from build123d import *

# Parameters (mm, degrees)
SKETCH_1_W             = 250
SKETCH_1_H             = 750
EXTRUDE_1_DEPTH        = 16
CUT_EXTRUDE_2_DEPTH    = 20
SKETCH_5_R             = 6.5
CUT_EXTRUDE_3_DEPTH    = 791.731307082
PATTERN_LINEAR_1_COUNT = 5
PATTERN_LINEAR_1_PITCH = 50
SKETCH_6_R             = 28
CUT_EXTRUDE_4_DEPTH    = 791.731307082
FILLET_1_R             = 60
SKETCH_7_W             = 250
SKETCH_7_H             = 40
CUT_EXTRUDE_5_DEPTH    = 66


with BuildPart() as part:
    # 草图1 → 凸台-拉伸1 (new body)
    with BuildSketch(Plane(origin=(0, 0, 0), x_dir=(0, 0, -1), z_dir=(1, 0, 0))):
        with Locations((125, 375)):
            Rectangle(SKETCH_1_W, SKETCH_1_H)
    extrude(amount=EXTRUDE_1_DEPTH)

    # 草图3 → 切除-拉伸2 (cut)
    with BuildSketch(Plane.ZY):
        Polygon((-130, 0), (0, 250), (0, 0), align=None)
    extrude(amount=-CUT_EXTRUDE_2_DEPTH, mode=Mode.SUBTRACT)

    # 草图5 → 切除-拉伸3 (cut, through all)
    with BuildSketch(Plane.ZY):
        with Locations((-225, 665)):
            Circle(SKETCH_5_R)
        with Locations((-225, 505)):
            Circle(SKETCH_5_R)
        with Locations((-225, 485)):
            Circle(SKETCH_5_R)
    cut_extrude_3 = extrude(amount=-CUT_EXTRUDE_3_DEPTH, mode=Mode.SUBTRACT)

    # 阵列(线性)1: 切除-拉伸3 ×5
    with Locations(*[(0, 0, i * PATTERN_LINEAR_1_PITCH) for i in range(1, PATTERN_LINEAR_1_COUNT)]):
        add(cut_extrude_3, mode=Mode.SUBTRACT)

    # 草图6 → 切除-拉伸4 (cut, through all)
    with BuildSketch(Plane.ZY):
        with Locations((-140, 105)):
            Circle(SKETCH_6_R)
    extrude(amount=-CUT_EXTRUDE_4_DEPTH, mode=Mode.SUBTRACT)

    # 圆角1
    fillet_1_edges = [part.edges().sort_by_distance(p)[0] for p in [
        (8, 0, -130),
        (8, 250, 0),
    ]]
    fillet(fillet_1_edges, radius=FILLET_1_R)

    # 草图7 → 切除-拉伸5 (cut)
    with BuildSketch(Plane(origin=(16, 0, 0), x_dir=(0, 0, -1), z_dir=(1, 0, 0))):
        with Locations((125, 730)):
            Rectangle(SKETCH_7_W, SKETCH_7_H)
    extrude(amount=-CUT_EXTRUDE_5_DEPTH, mode=Mode.SUBTRACT)


solid = part.part
Check sheet for the modelled part. Datum: model origin and axes. Units: mm. Coordinates: 2 decimals unless noted, no trailing zeros. Loops run counter-clockwise (first coordinate to the right, second up) from the corner with the lowest first, then second, coordinate; pieces in that order, holes last. Notation, with made-up numbers: (59, 87) -> (101, 87) arc R28 ccw to (101, 123) -> close; hole circle Ø3 at (57.25, 18). An arc over 180 degrees is marked (long way). Answer in a Markdown table with one row per item.
1. Sectioned sample at D-D, the plane z = -25. Record the boundary of the cut face in (x, y).
Check values:
| item | result |
|---|---|
| outline | (0, 201.92) -> (16, 201.92) -> (16, 478.5) -> (0, 478.5) -> close; (0, 491.5) -> (16, 491.5) -> (16, 498.5) -> (0, 498.5) -> close; (0, 511.5) -> (16, 511.5) -> (16, 658.5) -> (0, 658.5) -> close; (0, 671.5) -> (16, 671.5) -> (16, 710) -> (0, 710) -> close |
2. Release check for a two-part mould opening along Z. For faces 1 (the face through (8.112, 250.615, -1.669)), 2 (the face through (0, 360, -123)), 3 (the face through (7.888, 659.233, -72.001)) record: released by +Z, released by -Z, zero draft, split by the parting line, or undercut.
Check values:
| item | result |
|---|---|
| face 1 | released by +Z |
| face 2 | zero draft |
| face 3 | undercut |
3. Sectioned sample at B-B, the plane x = 3.75. Give the number of separate pieces and of enclosed holes in the cut face, then the cut area to 3 significant figures.
Check values:
| item | result |
|---|---|
| separate pieces | 1 |
| enclosed holes | 16 |
| area | 157,000 mm2 |
4. Sectioned sample at C-C, the plane y = 665. Record the boundary of the cut face in (x, z), then the cut area to 3 significant figures.
Check values:
| item | result |
|---|---|
| outline | (0, -250) -> (16, -250) -> (16, -231.5) -> (0, -231.5) -> close; (0, -218.5) -> (16, -218.5) -> (16, -181.5) -> (0, -181.5) -> close; (0, -168.5) -> (16, -168.5) -> (16, -131.5) -> (0, -131.5) -> close; (0, -118.5) -> (16, -118.5) -> (16, -81.5) -> (0, -81.5) -> close; (0, -68.5) -> (16, -68.5) -> (16, -31.5) -> (0, -31.5) -> close; (0, -18.5) -> (16, -18.5) -> (16, 0) -> (0, 0) -> close |
| area | 2,960 mm2 |
5. Material ranges on line 1 along Z through (x, y) = (11.5, 665); line 2 along Y through (x, z) = (11.25, -175); line 3 along Y through (x, z) = (5, -25), recorded low to high. Write a range as [from, to].
Check values:
| item | result |
|---|---|
| line 1 | z = [-250, -231.5], [-218.5, -181.5], [-168.5, -131.5], [-118.5, -81.5], [-68.5, -31.5], [-18.5, 0] |
| line 2 | y = [0, 478.5], [491.5, 498.5], [511.5, 658.5], [671.5, 710] |
| line 3 | y = [201.92, 478.5], [491.5, 498.5], [511.5, 658.5], [671.5, 710] |
6. Sectioned sample at A-A, the plane y = 105. Record the boundary of the cut face in (x, z).
Check values:
| item | result |
|---|---|
| outline | (0, -250) -> (16, -250) -> (16, -168) -> (0, -168) -> close; (0, -112) -> (16, -112) -> (16, -75.4) -> (0, -75.4) -> close |
7. Go/stop test with flat-tipped pins: pin 1 (10.5 mm diameter, centred on y = 505, z = -225, fed in from -X); pin 2 (2 mm diameter, centred on x = 7.5, y = 182.5, fed in from +Z). Record where each tip stops, or that it passes through.
Check values:
| item | result |
|---|---|
| pin 1 | passes through |
| pin 2 | stops at z = -34.58 |
